```python
from build123d import *

# Parameters (mm, degrees)
F1_DEPTH = 13
F0_W     = 7.5
F0_H     = 2
F2_DEPTH = 2
F3_R     = 2


with BuildPart() as f1:
    # F0 (on Top) → F1 (new body)
    with BuildSketch(Plane.XY):
        Polygon((3.75, -3.25), (6.5, -3.25), (6.5, 3.25), (-6.5, 3.25), (-6.5, -3.25), (-3.75, -3.25), (-3.75, -1.25), (-4.5, -1.25), (-4.5, 1.25), (4.5, 1.25), (4.5, -1.25), (3.75, -1.25), align=None)
    extrude(amount=F1_DEPTH)

    # F0 (on Top) → F2 (join)
    with BuildSketch(Plane.XY):
        Polygon((3.75, -3.25), (6.5, -3.25), (6.5, 3.25), (-6.5, 3.25), (-6.5, -3.25), (-3.75, -3.25), (-3.75, -1.25), (-4.5, -1.25), (-4.5, 1.25), (4.5, 1.25), (4.5, -1.25), (3.75, -1.25), align=None)
        Polygon((-3.75, -1.25), (3.75, -1.25), (4.5, -1.25), (4.5, 1.25), (-4.5, 1.25), (-4.5, -1.25), align=None)
        with Locations((0, -2.25)):
            Rectangle(F0_W, F0_H)
    extrude(amount=F2_DEPTH)

    # F3
    f3_edges = [f1.edges().sort_by_distance(p)[0] for p in [
        (-6.5, -3.25, 6.5),
        (6.5, -3.25, 6.5),
    ]]
    fillet(f3_edges, radius=F3_R)


solid = f1.part
```
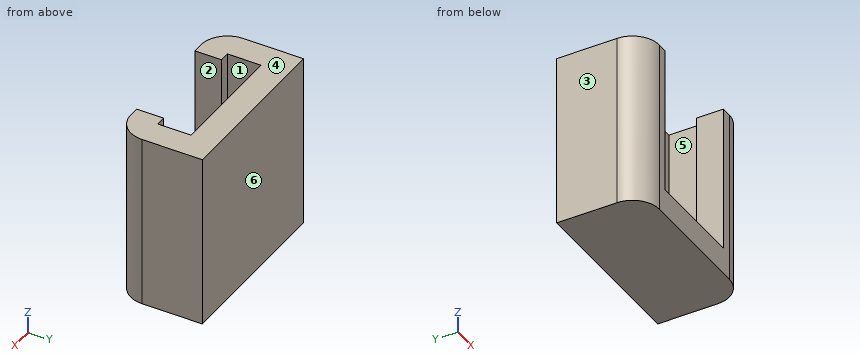
For this review, take the finished solid that the model builds, in its own axes (mm). Face numbers are marked on the shaded views. A direction names the side the tool comes from. Round coordinates to 2 decimals unless told otherwise and drop trailing zeros. Write each loop counter-clockwise with the first axis right and the second up, starting at its lowest first coordinate (ties: lowest second). Pieces come first, ordered by that corner, then holes. Notation, with made-up numbers: (-21.5, 37) -> (29.5, 37) arc R10 ccw to (29.5, 53) -> close; hole circle Ø8 at (1, 28). An arc over 180 degrees is marked (long way). Use one line per item in the form item = value.
Q1. To check wall thickness, follow probe 1 along X at (y, z) = (-1, 4); probe 2 along Y at (x, z) = (1.5, 4.75); probe 3 along Z at (x, y) = (3, -3). State the ranges of each line that lie inside material, in increasing order. Write a range as from..to.
Resolved:
probe_1 = -6.5..-4.5, 4.5..6.5
probe_2 = 1.25..3.25
probe_3 = 0..2
Q2. The part is to be moulded in two halves that separate along Y. For the marked faces 4, 5 and 6, say which applies: released by +Y, released by -Y, zero draft, split by the parting line, or undercut.
Resolved:
face_4 = zero draft
face_5 = undercut
face_6 = released by +Y
Q3. Machinability: for the marked faces 1, 2 and 3, which of the approach directions +Z, -Z, +X, -X, +Y, -Y give a long, thin tool a straight path to every point of the face, cutting with its end or side? Answer none if there is none.
Resolved:
face_1 = +Z
face_2 = +Z, -Y
face_3 = +Z, -Z, -X, +Y, -Y
Q4. Clearance check with flat-ended pins moving along their axes: pin 1 Ø2 at (x, y) = (-0.5, -1) entering from +Z; pin 2 Ø0.6 at (y, z) = (-2.5, 8.5) entering from -X; pin 3 Ø2.5 at (x, z) = (-1.5, 6.5) entering from -Y. State where each tip first meets the part, or that it passes through.
Resolved:
pin_1 = 2
pin_2 = -6.26
pin_3 = 1.25
Q5. Consider section A-A (y = 1). State the section outline as (x, z) points, then the cut area to 3 significant figures.
Resolved:
outline = (-6.5, 0) -> (6.5, 0) -> (6.5, 13) -> (4.5, 13) -> (4.5, 2) -> (-4.5, 2) -> (-4.5, 13) -> (-6.5, 13) -> close
area = 70.0 mm²
Q6. Consider section B-B (z = 9). State the section outline as (x, y) points, then the cut area to 3 significant figures.
Resolved:
outline = (-6.5, -1.25) arc R2 ccw to (-4.5, -3.25) -> (-3.75, -3.25) -> (-3.75, -1.25) -> (-4.5, -1.25) -> (-4.5, 1.25) -> (4.5, 1.25) -> (4.5, -1.25) -> (3.75, -1.25) -> (3.75, -3.25) -> (4.5, -3.25) arc R2 ccw to (6.5, -1.25) -> (6.5, 3.25) -> (-6.5, 3.25) -> close
area = 45.3 mm²
Q7. Consider section C-C (x = 0.75). State the section outline as (y, z) points, then the cut area to 3 significant figures.
Resolved:
outline = (-3.25, 0) -> (3.25, 0) -> (3.25, 13) -> (1.25, 13) -> (1.25, 2) -> (-3.25, 2) -> close
area = 35.0 mm²
Q8. Consider section D-D (y = -3). State the section outline as (x, z) points.
Resolved:
outline = (-5.47, 0) -> (5.47, 0) -> (5.47, 13) -> (3.75, 13) -> (3.75, 2) -> (-3.75, 2) -> (-3.75, 13) -> (-5.47, 13) -> close
